Verification items for the finished model (mm, model axes). A direction names the side the tool comes from. Coordinates: 2 decimals unless noted, no trailing zeros. Order: outer loops, then holes, each group sorted by start corner. A loop starts at its lowest first (then second) coordinate and runs counter-clockwise, first axis right, second up. Notation, with made-up numbers: M -5.5,84.25 L 39.5,84.25 A19 ccw 39.5,106.25 Z; hole C -22,73 d10. An arc over 180 degrees is marked long. Return JSON: item names as keys, results as strings.
```python
from build123d import *

# Parameters (mm, degrees)
CROQUIS1_R                   = 1.5
SALIENTE_EXTRUIR1_DEPTH      = 7
SALIENTE_EXTRUIR3_DEPTH      = 21
SALIENTE_EXTRUIR3_DEPTH_BACK = 3
CROQUIS3_R                   = 2.35


with BuildPart() as part:
    # Croquis1 → Saliente-Extruir1 (new body)
    with BuildSketch(Plane(origin=(0, 0, 0), x_dir=(1, 0, 0), z_dir=(0, 1, 0))):
        with BuildLine():
            Line((12.967669222, -4), (-12.4902, -4))
            ThreePointArc((-12.4902, -4), (-18.53478474, -3.968671916), (-20.133802427, 1.860661543))
            Line((-20.133802427, 1.860661543), (-21.263589404, 6.064668523))
            ThreePointArc((-21.263589404, 6.064668523), (-21.68376794, 13.566277491), (-14.19064257, 13.015133868))
            Line((-14.19064257, 13.015133868), (13.709196644, 4.992255837))
            ThreePointArc((13.709196644, 4.992255837), (20.470001725, -0.091961868), (12.967669222, -4))
        make_face()
        with Locations(Location((-15.491842215, 0, 0), (0, 0, 270))):
            Circle(CROQUIS1_R, mode=Mode.SUBTRACT)
        with Locations(Location((15.486915831, 0.318957805, 0), (0, 0, 90))):
            Circle(CROQUIS1_R, mode=Mode.SUBTRACT)
    extrude(amount=SALIENTE_EXTRUIR1_DEPTH)

    # Croquis3 → Saliente-Extruir3 (add, two sides: drawn at the far end of the back side and taken through both)
    with BuildSketch(Plane(origin=(-5.028546726, 0, -18.711532324), x_dir=(-0.9657345126344663, 0, 0.25953198474690947), z_dir=(-0.2595319847469094, 0, -0.9657345126344662)).offset(-SALIENTE_EXTRUIR3_DEPTH_BACK)):
        with Locations((14.961006691, 3.5)):
            Circle(CROQUIS3_R)
    extrude(amount=SALIENTE_EXTRUIR3_DEPTH + SALIENTE_EXTRUIR3_DEPTH_BACK)


solid = part.part
```
Q1. Go/stop test with flat-tipped pins: pin 1 (1.5 mm diameter, centred on x = -13.5, y = 2.5, fed in from -Z); pin 2 (3.5 mm diameter, centred on x = -1, y = 4.5, fed in from +Z). Record where each tip stops, or that it passes through.
Values:
{"pin 1": "z = -13.09", "pin 2": "z = 4"}
Q2. Tool access check on faces 4 (the face through (0, 3, 4)), 5 (the face through (-14.005, 3.451, -0.195)), 6 (the face through (-20.69, 3.45, -3.93)). Record the directions out of +Z, -Z, +X, -X, +Y, -Y that give a thin tool (end or side, any length) a straight path to the whole face; none if there is none.
Values:
{"face 4": "+Z, +Y, -Y", "face 5": "+Y, -Y", "face 6": "-X, +Y, -Y"}
Q3. Cross-section at A-A, the plane y = 2.25. Record the boundary of the cut face in (x, z).
Values:
{"outline": "M -26.85,-34.59 L -23.01,-35.63 L -17.45,-14.95 A5 ccw -14.19,-13.02 L 13.71,-4.99 A5 ccw long 12.97,4 L -12.49,4 A5 ccw -20.13,-1.86 L -21.26,-6.06 A5 ccw -21.29,-13.91 Z; hole C -15.49,0 d3; hole C 15.49,-0.32 d3"}
Q4. Cross-section at B-B, the plane z = 0. Record the boundary of the cut face in (x, y), and give its area (3 significant figures).
Values:
{"outline": "M -20.49,0 L -16.99,0 L -16.99,7 L -20.49,7 Z; M -13.99,0 L 14.02,0 L 14.02,7 L -13.99,7 Z; M 16.95,0 L 20.48,0 L 20.48,7 L 16.95,7 Z", "area": "245 mm^2"}
Q5. Draft check along X on faces 1 (the face through (-24.895, 3.533, -35.118)), 2 (the face through (16.95, 3.45, 0.01)), 3 (the face through (-24.183, 2.6, -23.976)). Enter one of: pulls with the +X half, pulls with the -X half, needs draft (parallel to the pull), parting line crosses it, or undercut.
Values:
{"face 1": "pulls with the -X half", "face 2": "undercut", "face 3": "parting line crosses it"}
Q6. Cross-section at C-C, the plane y = 5. Record the boundary of the cut face in (x, z).
Values:
{"outline": "M -26.67,-34.64 L -23.18,-35.58 L -17.64,-14.97 A5 ccw -14.19,-13.02 L 13.71,-4.99 A5 ccw long 12.97,4 L -12.49,4 A5 ccw -20.13,-1.86 L -21.26,-6.06 A5 ccw -21.14,-14.03 Z; hole C -15.49,0 d3; hole C 15.49,-0.32 d3"}
Q7. Cross-section at D-D, the plane x = -5. Record the boundary of the cut face in (y, z), and give its area (3 significant figures).
Values:
{"outline": "M 0,-10.37 L 7,-10.37 L 7,4 L 0,4 Z", "area": "101 mm^2"}
Q8. Material ranges on line 1 along X through (y, z) = (1.5, 1); line 2 along Z through (x, y) = (10, 5.5); line 3 along X through (y, z) = (4.75, -1), recorded low to high.
Values:
{"line 1": "-20.39 to -16.61, -14.37 to 14.77, 16.2 to 20.31", "line 2": "-6.06 to 4", "line 3": "-20.39 to -16.61, -14.37 to 14.15, 16.82 to 20.44"}
